Could you check a few things on this model? Use its own coordinates, in mm. A direction names the side the tool comes from. Coordinates: 2 decimals unless noted, no trailing zeros. Write each loop counter-clockwise with the first axis right and the second up, starting at its lowest first coordinate (ties: lowest second). Pieces come first, ordered by that corner, then holes.
Item 1: For P1, Ø8.5, axis at x = 14, z = 9.5, coming from the -Y side; P2, Ø3, axis at x = 25.5, z = 90, coming from the -Y side; P3, Ø4, axis at y = -13.5, z = 96, coming from the +X side; P4, Ø4, axis at x = 15, y = -10, coming from the -Z side, each with a flat end and sliding along its axis, tell me the tip position at first contact or that it passes through.
Item 2: Which directions (+Z, -Z, +X, -X, +Y, -Y) give clear straight access to the entire face, cutting with the end or side of a thin tool? Please do faces 4 (the flat face through (15, 0, 101)), 5 (the cylindrical face through (26.99, -17.15, 109.04)).
Item 3: I want a section at D-D on x = 22.25. Please give me the cut outline in (y, z).
Item 4: Thinking about a two-plate mould opening in Z: for faces 1 (the flat face through (15, -5, 0)), 2 (the flat face through (18, -10, 106.5)), 3 (the cylindrical face through (13.9, -12.11, 2.47)), which applies, +Z half, -Z half, draft (parallel to the pull), parting line (faces both ways), or undercut?
Item 5: I want a section at C-C on z = 45. Please give me the cut outline in (x, y).
Item 6: I want a section at A-A on x = 15. State how many separate pieces and enclosed holes the cut face has, then the cut area to 3 significant figures.
Item 7: I want a section at B-B on y = -14.75. Please give me the cut outline in (x, z).
Item 8: If I drill on probe 1 along Z at (x, y) = (26, -14.75); probe 2 along Y at (x, z) = (15, 107.8); probe 3 along Y at (x, z) = (9.25, 75.5), over which ranges is the centre line in solid material (lowest first)?
from build123d import *

# Parameters (mm, degrees)
ESQUISSE1_W                             = 30
ESQUISSE1_H                             = 10
BOSS_EXTRU_1_DEPTH                      = 111.5
ESQUISSE2_W                             = 30
ESQUISSE2_H                             = 5
BOSS_EXTRU_2_DEPTH                      = 20
PER_AGE_POUR_CROUS_AUTO_BLOQUANTS_300_D = 4.7625
CONG_1_R                                = 10


with BuildPart() as part:
    # Esquisse1 → Boss.-Extru.1 (new body)
    with BuildSketch(Plane.XY):
        with Locations((15, 5)):
            Rectangle(ESQUISSE1_W, ESQUISSE1_H)
    extrude(amount=BOSS_EXTRU_1_DEPTH)

    # Esquisse2 → Boss.-Extru.2 (add)
    with BuildSketch(Plane.XZ):
        with Locations((15, 2.5)):
            Rectangle(ESQUISSE2_W, ESQUISSE2_H)
        with Locations((15, 18)):
            Rectangle(ESQUISSE2_W, ESQUISSE2_H)
        with Locations((15, 109)):
            Rectangle(ESQUISSE2_W, ESQUISSE2_H)
        with Locations((15, 93.5)):
            Rectangle(ESQUISSE2_W, ESQUISSE2_H)
    extrude(amount=BOSS_EXTRU_2_DEPTH)

    # Perçage pour écrous auto-bloquants 300® #6 (SP)1 (through all)
    with Locations(Plane.XY.offset(111.5)):
        with Locations((15, -10)):
            Hole(PER_AGE_POUR_CROUS_AUTO_BLOQUANTS_300_D / 2)

    # Congé1
    cong_1_edges = [part.edges().sort_by_distance(p)[0] for p in [
        (0, -20, 2.5),
        (30, -20, 2.5),
        (30, -20, 18),
        (0, -20, 18),
        (0, -20, 109),
        (30, -20, 109),
        (30, -20, 93.5),
        (0, -20, 93.5),
    ]]
    fillet(cong_1_edges, radius=CONG_1_R)


solid = part.part
Response values:
1. P1: stops at y = 0
1. P2: stops at y = -18.99
1. P3: stops at x = 29.89
1. P4: passes through
2. face 4: +X, -X, -Y
2. face 5: +Z, -Z, +X, -Y
3. outline: (-19.74, 0) - (10, 0) - (10, 111.5) - (-19.74, 111.5) - (-19.74, 106.5) - (0, 106.5) - (0, 96) - (-19.74, 96) - (-19.74, 91) - (0, 91) - (0, 20.5) - (-19.74, 20.5) - (-19.74, 15.5) - (0, 15.5) - (0, 5) - (-19.74, 5) - close
4. face 1: -Z half
4. face 2: undercut
4. face 3: draft
5. outline: (0, 0) - (30, 0) - (30, 10) - (0, 10) - close
6. separate pieces: 5
6. enclosed holes: 0
6. area: 1,420 mm2
7. outline: (1.2, 0) - (28.8, 0) - (28.8, 5) - (1.2, 5) - close; (1.2, 15.5) - (28.8, 15.5) - (28.8, 20.5) - (1.2, 20.5) - close; (1.2, 91) - (28.8, 91) - (28.8, 96) - (1.2, 96) - close; (1.2, 106.5) - (28.8, 106.5) - (28.8, 111.5) - (1.2, 111.5) - close
8. probe 1: z = 0 to 5, 15.5 to 20.5, 91 to 96, 106.5 to 111.5
8. probe 2: y = -20 to -12.38, -7.62 to 10
8. probe 3: y = 0 to 10
